For this review, use the dimensioned drawing (mm, ordinates from the lowest corner) and the shaded views. A direction names the side the tool comes from. Coordinates: 2 decimals unless noted, no trailing zeros. Write each loop counter-clockwise with the first axis right and the second up, starting at its lowest first coordinate (ties: lowest second). Pieces come first, ordered by that corner, then holes. Notation, with made-up numbers: (67, -35) - (79, -35) arc R17 ccw to (79, -7) - close; hole circle Ø2 at (-18.5, -2.75). An arc over 180 degrees is marked (long way). Use one line per item in the form item = value. Start each with the question number.
1) Tool access review of the marked faces 4, 5 and 6: name each direction out of +Z, -Z, +X, -X, +Y, -Y from which nothing blocks a thin tool from reaching the whole face with its end or side.
2) We need section B-B (y = 12.5). Give the boundary of the cut face in (x, z).
3) For L1, parallel to X at y = 16.3, z = 9.5; L2, parallel to X at y = 19, z = 5.75; L3, parallel to Y at x = 58, z = 14.4, list the stretches that pass through material, from the lowest coordinate up. Write a range as from..to.
4) We need section A-A (x = 5). Give the boundary of the cut face in (y, z), plus the area to 3 significant figures.
5) Mouldability with a two-part tool opening along X and no side actions: class the marked faces 1, 2 and 3 as pulls with the +X half, pulls with the -X half, needs draft (parallel to the pull), parting line crosses it, or undercut.
6) Insertion check: P1, Ø4.5, axis at x = 56, z = 13.5, coming from the +Y side; P2, Ø4, axis at y = 14.5, z = 11, coming from the +X side; P3, Ø5, axis at x = 9, y = 7.5, coming from the -Z side; P4, Ø1.6, axis at x = 17.6, z = 9.5, coming from the -Y side. Each pin has a flat end and moves straight along its axis. Give the tip position at first contact, or say it passes through.
7) We need section D-D (z = 14). Give the boundary of the cut face in (x, y), plus the area to 3 significant figures.
8) We need section C-C (z = 9.5). Give the boundary of the cut face in (x, y), plus the area to 3 significant figures.
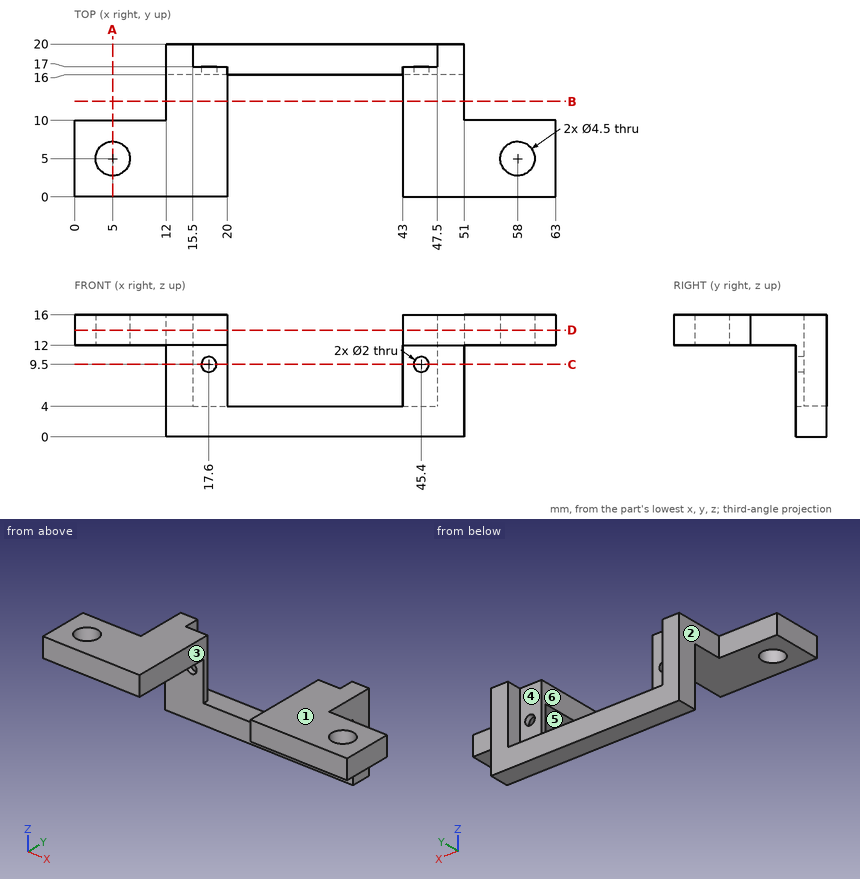
Determined:
q1.face_4 = +Z, +Y
q1.face_5 = -Z, +X, -X, -Y
q1.face_6 = +Z, +Y, -Y
q2.outline = (12, 12) - (20, 12) - (20, 16) - (12, 16) - close; (43, 12) - (51, 12) - (51, 16) - (43, 16) - close
q3.L1 = 12..16.6, 18.6..20, 43..44.4, 46.4..51
q3.L2 = 12..15.5, 47.5..51
q3.L3 = 0..2.75, 7.25..10
q4.outline = (0, 12) - (2.75, 12) - (2.75, 16) - (0, 16) - close; (7.25, 12) - (10, 12) - (10, 16) - (7.25, 16) - close
q4.area = 22.0 mm²
q5.face_1 = needs draft
q5.face_2 = pulls with the -X half
q5.face_3 = undercut
q6.P1 = 10
q6.P2 = 51
q6.P3 = 12
q6.P4 = through
q7.outline = (0, 0) - (20, 0) - (20, 17) - (15.5, 17) - (15.5, 20) - (12, 20) - (12, 10) - (0, 10) - close; (43, 0) - (63, 0) - (63, 10) - (51, 10) - (51, 20) - (47.5, 20) - (47.5, 17) - (43, 17) - close; hole circle Ø4.5 at (5, 5); hole circle Ø4.5 at (58, 5)
q7.area = 501 mm²
q8.outline = (12, 16) - (16.6, 16) - (16.6, 17) - (15.5, 17) - (15.5, 20) - (12, 20) - close; (18.6, 16) - (20, 16) - (20, 17) - (18.6, 17) - close; (43, 16) - (44.4, 16) - (44.4, 17) - (43, 17) - close; (46.4, 16) - (51, 16) - (51, 20) - (47.5, 20) - (47.5, 17) - (46.4, 17) - close
q8.area = 33.0 mm²
